Part model, mm, in its own coordinate system. Face numbers are marked on the shaded views. Give positions to 0.01 mm unless a question says otherwise; leave off trailing zeros. Write each loop counter-clockwise with the first axis right and the second up, starting at its lowest first coordinate (ties: lowest second). Pieces come first, ordered by that corner, then holes.
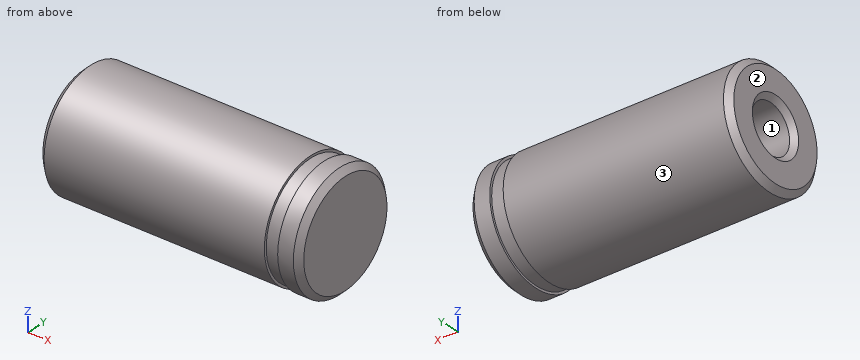
Autodesk Inventor part; units mm, degrees
ref_plane "to_ring_F_R_XY" through (20.075, 0, 0) normal (1, 0, 0) x (0, 0, -1)
ref_plane "to_ring_F_R_YZ" through (20.075, 0, 0) normal (0, 0, -1) x (0, 1, 0)
ref_plane "to_ring_F_R_ZX" through (20.075, 0, 0) normal (0, 1, 0) x (1, 0, 0)
sketch "Sketch_1" plane through (0, 0, 0) normal (0, 0, 1) x (1, 0, 0)
  line L0 (22.5, 0) -> (0, 0)
  line L1 (0, 0) -> (0, 4.5)
  line L2 (0, 4.5) -> (0.5, 5)
  line L3 (0.5, 5) -> (22, 5)
  line L4 (22, 5) -> (22.5, 4.5)
  line L5 (22.5, 4.5) -> (22.5, 0)
  line L6 (22.5, 0) -> (0, 0)
revolve "Revolution1" add sketch "Sketch_1" angle 360 about axis through (22.5, 0, 0) along (1, 0, 0)
sketch "Sketch2" plane through (0, 0, 0) normal (-1, 0, 0) x (0, 0, 1)
  point P0 (0, 0)
hole "Hole1" at (0, 0, 0) direction (1, 0, 0) diameter 4.134 depth 13.8066 tip angle 120 countersink diameter 5 countersink angle 90
sketch "Sketch_20" plane through (0, 0, 0) normal (0, 0, 1) x (1, 0, 0)
  line L0 (22.5, 0) -> (-22.5, 0)
  line L1 (19.5, 9.6) -> (19.5, 4.8)
  line L2 (19.5, 4.8) -> (20.65, 4.8)
  line L3 (20.65, 4.8) -> (20.65, 9.6)
  line L4 (20.65, 9.6) -> (19.5, 9.6)
revolve "Revolution2" cut sketch "Sketch_20" angle 360 about axis through (22.5, 0, 0) along (1, 0, 0)
ref_plane "to_ring_F_R_XY" through (20.075, 0, 0) normal (1, 0, 0) x (0, 0, -1)
ref_plane "to_ring_F_R_YZ" through (20.075, 0, 0) normal (0, 0, -1) x (0, 1, 0)
ref_plane "to_ring_F_R_ZX" through (20.075, 0, 0) normal (0, 1, 0) x (1, 0, 0)
properties part number "SSFRBF-D10-L22.5-M5-U3"
1) Saw through at B-B, the plane x = 9.75. Write the cut outline in (y, z).
Answers follow:
outline: circle Ø10 at (0, 0); hole circle Ø4.13 at (0, 0)
2) Wall check: L1, parallel to Z at x = 8.5, y = 0; L2, parallel to Z at x = 11.5, y = 1.5; L3, parallel to Z at x = 14.25, y = -2. Give the ranges that are in metal, low to high.
Answers follow:
L1: z = -5 to -2.07, 2.07 to 5
L2: z = -4.77 to -1.42, 1.42 to 4.77
L3: z = -4.58 to 4.58
3) Pin check, flat tips, straight feed: pin 1 Ø3 at (x, y) = (9.5, -1) entering from +Z; pin 2 Ø2 at (x, y) = (13.5, 2.5) entering from +Z. Stop position of each tip, or through.
Answers follow:
pin 1: stops at z = 5
pin 2: stops at z = 4.77
4) Two-plate mould, pull along Y, no slides. Class the marked faces 1, 2 and 3: +Y half, -Y half, draft (parallel to the pull), parting line (faces both ways), or undercut.
Answers follow:
face 1: undercut
face 2: draft
face 3: parting line
5) Saw through at A-A, the plane x = 17.25. Write the cut outline in (y, z), then the cut area to 3 significant figures.
Answers follow:
outline: circle Ø10 at (0, 0)
area: 78.5 mm2
